Part model, mm, in its own coordinate system. Give positions to 0.01 mm unless a question says otherwise; leave off trailing zeros. Order: outer loops, then holes, each group sorted by start corner. A loop starts at its lowest first (then second) coordinate and runs counter-clockwise, first axis right, second up. Notation, with made-up numbers: (-5, 36.25) - (37, 36.25) arc R7 cw to (37, 46.25) - close; hole circle Ø11 at (23.25, 51). An arc over 180 degrees is marked (long way). One line per item, written item: value.
```python
from build123d import *

# Parameters (mm, degrees)
SKETCH1_W           = 85
SKETCH1_H           = 138
BOSS_EXTRUDE1_DEPTH = 51.5
CUT_EXTRUDE2_REACH  = 87
SKETCH3_R           = 14.3
SKETCH3_R_2         = 15.83


with BuildPart() as part:
    # Sketch1 → Boss-Extrude1 (new body)
    with BuildSketch(Plane(origin=(0, 0, 0), x_dir=(1, 0, 0), z_dir=(0, 1, 0))):
        with Locations((42.5, 69)):
            Rectangle(SKETCH1_W, SKETCH1_H)
    extrude(amount=BOSS_EXTRUDE1_DEPTH)

    # Sketch3 → Cut-Extrude2 (cut, up to next)
    with BuildSketch(Plane(origin=(85, 0, 0), x_dir=(0, 0, -1), z_dir=(1, 0, 0)), mode=Mode.PRIVATE) as cut_extrude2_sk1:
        with Locations((69, 25.75)):
            Circle(SKETCH3_R)
    cut_extrude2_tool1 = extrude(cut_extrude2_sk1.sketch, amount=-CUT_EXTRUDE2_REACH, mode=Mode.PRIVATE) & part.part
    add(cut_extrude2_tool1.solids().sort_by_distance((85, 25.75, -69))[0], mode=Mode.SUBTRACT)
    # Sketch3 → Cut-Extrude2 (cut, up to next)
    with BuildSketch(Plane(origin=(85, 0, 0), x_dir=(0, 0, -1), z_dir=(1, 0, 0)), mode=Mode.PRIVATE) as cut_extrude2_sk2:
        with Locations((26.5, 25.75)):
            Circle(SKETCH3_R_2)
    cut_extrude2_tool2 = extrude(cut_extrude2_sk2.sketch, amount=-CUT_EXTRUDE2_REACH, mode=Mode.PRIVATE) & part.part
    add(cut_extrude2_tool2.solids().sort_by_distance((85, 25.75, -26.5))[0], mode=Mode.SUBTRACT)
    # Sketch3 → Cut-Extrude2 (cut, up to next)
    with BuildSketch(Plane(origin=(85, 0, 0), x_dir=(0, 0, -1), z_dir=(1, 0, 0)), mode=Mode.PRIVATE) as cut_extrude2_sk3:
        with Locations((111.5, 25.75)):
            Circle(SKETCH3_R_2)
    cut_extrude2_tool3 = extrude(cut_extrude2_sk3.sketch, amount=-CUT_EXTRUDE2_REACH, mode=Mode.PRIVATE) & part.part
    add(cut_extrude2_tool3.solids().sort_by_distance((85, 25.75, -111.5))[0], mode=Mode.SUBTRACT)


solid = part.part
```
1) Drop flat-ended pins along their axis: P1, Ø1.5, axis at x = 69.5, z = -80, coming from the -Y side; P2, Ø4, axis at y = 14.5, z = -104, coming from the -X side. Give the stop position or say it passes through.
Answer:
P1: stops at y = 0
P2: passes through
2) Two-plate mould, pull along Z, no slides. Class faces 1 (the face through (43.1, 30.5, -41.6)), 2 (the face through (43.095, 26.379, -54.714)), 3 (the face through (42, 25, 0)), 4 (the face through (42, 25, -138)): pulls with the +Z half, pulls with the -Z half, needs draft (parallel to the pull), parting line crosses it, or undercut.
Answer:
face 1: undercut
face 2: undercut
face 3: pulls with the +Z half
face 4: pulls with the -Z half
3) Wall check: line 1 along Z through (x, y) = (59, 25); line 2 along Y through (x, z) = (7.5, -26); line 3 along Z through (x, y) = (37, 38). Give the ranges that are in metal, low to high. Write a range as [from, to].
Answer:
line 1: z = [-138, -127.31], [-95.69, -83.28], [-54.72, -42.31], [-10.69, 0]
line 2: y = [0, 9.93], [41.57, 51.5]
line 3: z = [-138, -121.53], [-101.47, -76.38], [-61.62, -36.53], [-16.47, 0]
4) Slice it at C-C on z = -69. Write the cut outline in (x, y), then the cut area to 3 significant figures.
Answer:
outline: (0, 0) - (85, 0) - (85, 11.45) - (0, 11.45) - close; (0, 40.05) - (85, 40.05) - (85, 51.5) - (0, 51.5) - close
area: 1,950 mm2
5) Slice it at D-D on z = -31. Write the cut outline in (x, y), then the cut area to 3 significant figures.
Answer:
outline: (0, 0) - (85, 0) - (85, 10.57) - (0, 10.57) - close; (0, 40.93) - (85, 40.93) - (85, 51.5) - (0, 51.5) - close
area: 1,800 mm2
6) Slice it at A-A on y = 25.75. Write the cut outline in (x, z).
Answer:
outline: (0, -138) - (85, -138) - (85, -127.33) - (0, -127.33) - close; (0, -95.67) - (85, -95.67) - (85, -83.3) - (0, -83.3) - close; (0, -54.7) - (85, -54.7) - (85, -42.33) - (0, -42.33) - close; (0, -10.67) - (85, -10.67) - (85, 0) - (0, 0) - close
7) Slice it at B-B on x = 14.5. Write the cut outline in (y, z), then the cut area to 3 significant figures.
Answer:
outline: (0, -138) - (51.5, -138) - (51.5, 0) - (0, 0) - close; hole circle Ø31.66 at (25.75, -111.5); hole circle Ø31.66 at (25.75, -26.5); hole circle Ø28.6 at (25.75, -69)
area: 4,890 mm2
